```python
from build123d import *

# Parameters (mm, degrees)
SKETCH1_R           = 2.5
BOSS_EXTRUDE1_DEPTH = 10
CUT_EXTRUDE1_START  = 5
CUT_EXTRUDE1_DEPTH  = 5
SKETCH4_R           = 2.5
SKETCH4_R_2         = 20
CUT_EXTRUDE2_DEPTH  = 241.282833344


with BuildPart() as part:
    # Sketch1 → Boss-Extrude1 (new body)
    with BuildSketch(Plane.XY):
        Polygon((0, 0), (132.8, 0), (132.8, 65), (83.664018374, 200), (0, 200), align=None)
        with Locations((115.1, 27)):
            Circle(SKETCH1_R, mode=Mode.SUBTRACT)
        with Locations((89.1, 27)):
            Circle(SKETCH1_R, mode=Mode.SUBTRACT)
        with Locations((115.1, 53)):
            Circle(SKETCH1_R, mode=Mode.SUBTRACT)
        with Locations((89.1, 53)):
            Circle(SKETCH1_R, mode=Mode.SUBTRACT)
        with Locations((17.7, 53)):
            Circle(SKETCH1_R, mode=Mode.SUBTRACT)
        with Locations((17.7, 27)):
            Circle(SKETCH1_R, mode=Mode.SUBTRACT)
        with Locations((43.7, 27)):
            Circle(SKETCH1_R, mode=Mode.SUBTRACT)
        with Locations((43.7, 53)):
            Circle(SKETCH1_R, mode=Mode.SUBTRACT)
        with Locations((59.91, 29.92)):
            Circle(SKETCH1_R, mode=Mode.SUBTRACT)
        with Locations((59.91, 9.92)):
            Circle(SKETCH1_R, mode=Mode.SUBTRACT)
    extrude(amount=BOSS_EXTRUDE1_DEPTH)

    # Sketch1_3 → Cut-Extrude1 (cut)
    with BuildSketch(Plane.XY.offset(CUT_EXTRUDE1_START)):
        Polygon((64.535, 29.92), (62.2225, 33.925367493), (57.5975, 33.925367493), (55.285, 29.92), (57.5975, 25.914632507), (62.2225, 25.914632507), align=None)
        Polygon((62.2225, 13.925367493), (64.535, 9.92), (62.2225, 5.914632507), (57.5975, 5.914632507), (55.285, 9.92), (57.5975, 13.925367493), align=None)
    extrude(amount=CUT_EXTRUDE1_DEPTH, mode=Mode.SUBTRACT)

    # Sketch4 → Cut-Extrude2 (cut, through all)
    with BuildSketch(Plane(origin=(0, 0, 0), x_dir=(-1, 0, 0), z_dir=(0, 0, -1))):
        with Locations((-15, 187.5)):
            Circle(SKETCH4_R)
        with Locations((-35, 187.5)):
            Circle(SKETCH4_R)
        with Locations((-35, 110)):
            Circle(SKETCH4_R)
        with Locations((-15, 110)):
            Circle(SKETCH4_R)
        with Locations((-57, 148.75)):
            Circle(SKETCH4_R_2)
        with Locations((-33.5, 172.25)):
            Circle(SKETCH4_R)
        with Locations((-33.5, 125.25)):
            Circle(SKETCH4_R)
        with Locations((-80.5, 125.25)):
            Circle(SKETCH4_R)
        with Locations((-80.5, 172.25)):
            Circle(SKETCH4_R)
    extrude(amount=-CUT_EXTRUDE2_DEPTH, mode=Mode.SUBTRACT)


solid = part.part
```
The model under review builds one solid part; all positions refer to its coordinate system, in mm. A direction names the side the tool comes from. Round coordinates to 2 decimals unless told otherwise and drop trailing zeros. Loops run counter-clockwise (first coordinate to the right, second up) from the corner with the lowest first, then second, coordinate; pieces in that order, holes last. Notation, with made-up numbers: (23.5, -9) - (62.5, -9) arc R20 ccw to (62.5, 25) - close; hole circle Ø4 at (54, -5). An arc over 180 degrees is marked (long way). Use a Markdown table: item, result. Add a question column.
Q1. Add section B-B (y = 53). State the section outline as (x, z) points, plus the area to 3 significant figures.
Q2. Add section C-C (y = 110). State the section outline as (x, z) points, plus the area to 3 significant figures.
Q3. Add section D-D (y = 148.75). State the section outline as (x, z) points, plus the area to 3 significant figures.
Q4. For probe 1 along Y at (x, z) = (17.7, 2.5); probe 2 along Y at (x, z) = (80.5, 3.5); probe 3 along X at (y, z) = (127, 3), list the stretches that pass through material, from the lowest coordinate up.
Q5. The part is to be moulded in two halves that separate along X. For faces 1 (the face through (0, 101, 5)), 2 (the face through (19.04, 29.11, 4.93)), 3 (the face through (65, 0, 5)), 4 (the face through (108.576, 131.555, 4.93)), say which applies: pulls with the +X half, pulls with the -X half, needs draft (parallel to the pull), parting line crosses it, or undercut.
Q6. Insertion check: pin 1 Ø4 at (x, y) = (61, 11.5) entering from +Z. The pin has a flat end and moves straight along its axis. Give the tip position at first contact, or say it passes through.
Q7. Add section A-A (x = 80.5). State the section outline as (y, z) points, plus the area to 3 significant figures.
Q8. Machinability: for faces 5 (the face through (56.457, 7.889, 7.465)), 6 (the face through (57.412, 30.03, 2.465)), which of the approach directions +Z, -Z, +X, -X, +Y, -Y give a long, thin tool a straight path to every point of the face, cutting with its end or side? Answer none if there is none.
Worked answers:
| question | item | result |
|---|---|---|
| 1 | outline | (0, 0) - (15.2, 0) - (15.2, 10) - (0, 10) - close; (20.2, 0) - (41.2, 0) - (41.2, 10) - (20.2, 10) - close; (46.2, 0) - (86.6, 0) - (86.6, 10) - (46.2, 10) - close; (91.6, 0) - (112.6, 0) - (112.6, 10) - (91.6, 10) - close; (117.6, 0) - (132.8, 0) - (132.8, 10) - (117.6, 10) - close |
| 1 | area | 1,130 mm² |
| 2 | outline | (0, 0) - (12.5, 0) - (12.5, 10) - (0, 10) - close; (17.5, 0) - (32.5, 0) - (32.5, 10) - (17.5, 10) - close; (37.5, 0) - (116.42, 0) - (116.42, 10) - (37.5, 10) - close |
| 2 | area | 1,060 mm² |
| 3 | outline | (0, 0) - (37, 0) - (37, 10) - (0, 10) - close; (77, 0) - (102.32, 0) - (102.32, 10) - (77, 10) - close |
| 3 | area | 623 mm² |
| 4 | probe 1 | 0 to 24.5, 29.5 to 50.5, 55.5 to 200 |
| 4 | probe 2 | 0 to 122.75, 127.75 to 169.75, 174.75 to 200 |
| 4 | probe 3 | 0 to 31.71, 35.29 to 78.71, 82.29 to 110.23 |
| 5 | face 1 | pulls with the -X half |
| 5 | face 2 | undercut |
| 5 | face 3 | needs draft |
| 5 | face 4 | pulls with the +X half |
| 6 | pin 1 | z = 5 |
| 7 | outline | (0, 0) - (122.75, 0) - (122.75, 10) - (0, 10) - close; (127.75, 0) - (169.75, 0) - (169.75, 10) - (127.75, 10) - close; (174.75, 0) - (200, 0) - (200, 10) - (174.75, 10) - close |
| 7 | area | 1,900 mm² |
| 8 | face 5 | +Z |
| 8 | face 6 | +Z, -Z |
